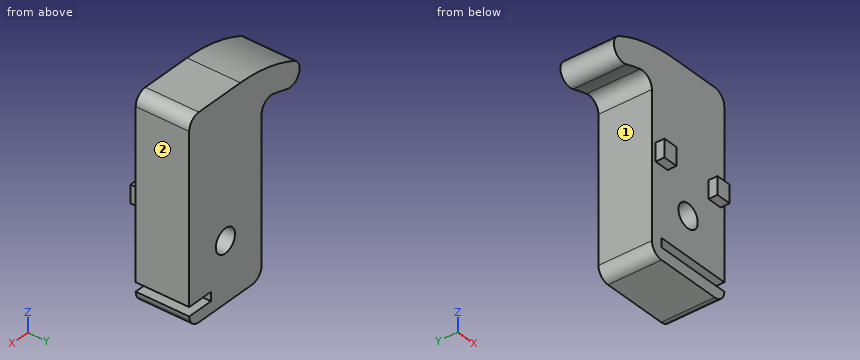
from build123d import *

# Parameters (mm, degrees)
SKETCH_1_R          = 2
EXTRUDE_1_DEPTH     = 9
SKETCH_3_W          = 2.5
SKETCH_3_H          = 3
EXTRUDE_2_DEPTH     = 1.5
CUT_EXTRUDE_1_REACH = 11
SKETCH_5_W          = 13
SKETCH_5_H          = 1.5
SKETCH_7_W          = 8.5
SKETCH_7_H          = 1.5
EXTRUDE_3_DEPTH     = 4
SKETCH_9_W          = 49.545975543
SKETCH_9_H          = 42.208236046
CUT_EXTRUDE_3_DEPTH = 11.5


with BuildPart() as part:
    # 草图1 → 凸台-拉伸1 (new body)
    with BuildSketch(Plane(origin=(0, 0, 0), x_dir=(1, 0, 0), z_dir=(0, 1, 0))):
        with BuildLine():
            Line((-2.382835885, 33.5), (8.617164115, 33.5))
            ThreePointArc((8.617164115, 33.5), (10.031377677, 32.914213562), (10.617164115, 31.5))
            Line((10.617164115, 31.5), (10.617164115, 2))
            ThreePointArc((10.617164115, 2), (10.031377677, 0.585786438), (8.617164115, 0))
            Line((8.617164115, 0), (0, 0))
            ThreePointArc((0, 0), (-5.710600422, 0.647655185), (-11.131122415, 2.557722132))
            ThreePointArc((-11.131122415, 2.557722132), (-12.111898361, 5.107720531), (-9.633282348, 6.257014206))
            ThreePointArc((-9.633282348, 6.257014206), (-8.243555708, 5.833986106), (-6.836394497, 5.473167269))
            ThreePointArc((-6.836394497, 5.473167269), (-5.139275919, 5.854675685), (-4.382835885, 7.421059613))
            Line((-4.382835885, 7.421059613), (-4.382835885, 31.5))
            ThreePointArc((-4.382835885, 31.5), (-3.797049447, 32.914213562), (-2.382835885, 33.5))
        make_face()
        with Locations((3.117164115, 23.5)):
            Circle(SKETCH_1_R, mode=Mode.SUBTRACT)
    extrude(amount=EXTRUDE_1_DEPTH)

    # 草图3 → 凸台-拉伸2 (add)
    with BuildSketch(Plane(origin=(0, 9, 0), x_dir=(1, 0, 0), z_dir=(0, 1, 0))):
        with Locations((-2.382835885, 17)):
            Rectangle(SKETCH_3_W, SKETCH_3_H)
        with Locations((8.617164115, 17)):
            Rectangle(SKETCH_3_W, SKETCH_3_H)
    extrude(amount=EXTRUDE_2_DEPTH)

    # 草图5 → 切除-拉伸1 (cut, up to next)
    with BuildSketch(Plane(origin=(0, 9, 0), x_dir=(1, 0, 0), z_dir=(0, 1, 0)), mode=Mode.PRIVATE) as cut_extrude_1_sk1:
        with Locations((4.117164115, 30.75)):
            Rectangle(SKETCH_5_W, SKETCH_5_H)
    cut_extrude_1_tool1 = extrude(cut_extrude_1_sk1.sketch, amount=-CUT_EXTRUDE_1_REACH, mode=Mode.PRIVATE) & part.part
    add(cut_extrude_1_tool1.solids().sort_by_distance((4.117164, 9, -30.75))[0], mode=Mode.SUBTRACT)

    # 草图7 → 凸台-拉伸3 (add)
    with BuildSketch(Plane.XZ):
        with Locations((1.867164115, -30.75)):
            Rectangle(SKETCH_7_W, SKETCH_7_H)
    extrude(amount=-EXTRUDE_3_DEPTH)

    # 镜向8: part across plane


with BuildPart() as part_1:
    add(part.part)
    add(part.part.mirror(Plane(origin=(0, 0, -25.5), x_dir=(0, 0, 1), z_dir=(0, -1, 0))))

    # 草图9 → 切除-拉伸3 (cut, through all)
    with BuildSketch(Plane(origin=(0, 0, 0), x_dir=(1, 0, 0), z_dir=(0, 1, 0))):
        with Locations((0.218507418, 15.905835279)):
            Rectangle(SKETCH_9_W, SKETCH_9_H)
    extrude(amount=CUT_EXTRUDE_3_DEPTH, mode=Mode.SUBTRACT)


solid = part_1.part
The listing builds one solid part. Answer for the finished solid, in the listing's coordinates (mm). Face numbers are marked on the shaded views. A direction names the side the tool comes from. Round coordinates to 2 decimals unless told otherwise and drop trailing zeros. Loops run counter-clockwise (first coordinate to the right, second up) from the corner with the lowest first, then second, coordinate; pieces in that order, holes last. Notation, with made-up numbers: M 54.25,-8.5 L 71.25,-8.5 A19 cw 71.25,24.5 Z; hole C 69.5,-10 d9. An arc over 180 degrees is marked long. Write each question's results on one line, items separated by ' | '. Start each with the question number.
1) Find section A-A on y = -6.25. Write down the section's boundary in (x, z), plus the area to 3 significant figures.
2) Find section C-C on x = 9.25. Write down the section's boundary in (y, z).
3) Which of the six approach directions +Z, -Z, +X, -X, +Y, -Y give full straight-line access (tool end or side, diameter ignored) to the marked faces 1 and 2?
4) Straight lines are drawn through the part: probe 1 along X at (y, z) = (-3.25, -23.5); probe 2 along Z at (x, y) = (6.5, -2); probe 3 along Y at (x, z) = (-5, -5.5). For each, find the intervals that lie inside material, in ascending order.
5) Each of these flat-tipped pins is pushed along its axis until it touches: pin 1 (1.6 mm diameter, centred on x = -2.5, y = -10, fed in from +Z); pin 2 (4 mm diameter, centred on x = -4, z = -6.5, fed in from -Y); pin 3 (5 mm diameter, centred on x = -8.5, y = -7, fed in from +Z). Where does it stop, or does it pass through?
6) Find section B-B on z = -23.5. Write down the section's boundary in (x, y), plus the area to 3 significant figures.
7) Find section D-D on x = 3. Write down the section's boundary in (y, z), plus the area to 3 significant figures.
Final values:
1) outline: M -11.13,-2.56 A2 ccw -9.63,-6.26 A32.66 cw -6.84,-5.47 A2 cw -4.38,-7.42 L -4.38,-31.5 A2 ccw -2.38,-33.5 L 8.62,-33.5 A2 ccw 10.62,-31.5 L -2.38,-31.5 L -2.38,-30 L 10.62,-30 L 10.62,-2 A2 ccw 8.62,0 L 0,0 A25.5 ccw Z; hole C 3.12,-23.5 d4 | area: 501 mm²
2) outline: M -10.5,-18.5 L -9,-18.5 L -9,-30 L 0,-30 L 0,-0.1 L -9,-0.1 L -9,-15.5 L -10.5,-15.5 Z; M -9,-33.4 L 0,-33.4 L 0,-31.5 L -9,-31.5 Z
3) face 1: -Z, -X, +Y, -Y | face 2: +Z, -Z, +X, +Y, -Y
4) probe 1: -4.38 to 1.12, 5.12 to 10.62 | probe 2: -33.5 to -31.5, -30 to 0 | probe 3: -9 to 0
5) pin 1: z = -15.5 | pin 2: y = -9 | pin 3: z = -0.72
6) outline: M -4.38,-9 L 1.12,-9 L 1.12,0 L -4.38,0 Z; M 5.12,-9 L 10.62,-9 L 10.62,0 L 5.12,0 Z | area: 99.0 mm²
7) outline: M -9,-33.5 L 0,-33.5 L 0,-25.5 L -9,-25.5 L -9,-30 L -4,-30 L -4,-31.5 L -9,-31.5 Z; M -9,-21.5 L 0,-21.5 L 0,0 L -9,0 Z | area: 258 mm²
